Geometry: see drawing. Coordinates: mm, zero at the bounding-box minimum. A direction names the side the tool comes from. Give positions to 0.01 mm unless a question says otherwise; leave off trailing zeros. Order: outer loops, then holes, each group sorted by start corner. A loop starts at its lowest first (then second) coordinate and runs counter-clockwise, first axis right, second up. Notation, with made-up numbers: (-15.5, 67.25) - (15.5, 67.25) arc R19 ccw to (15.5, 87.25) - close; hole circle Ø3 at (22.5, 20). An arc over 180 degrees is marked (long way). One line per item, written item: value. Start each with the question number.
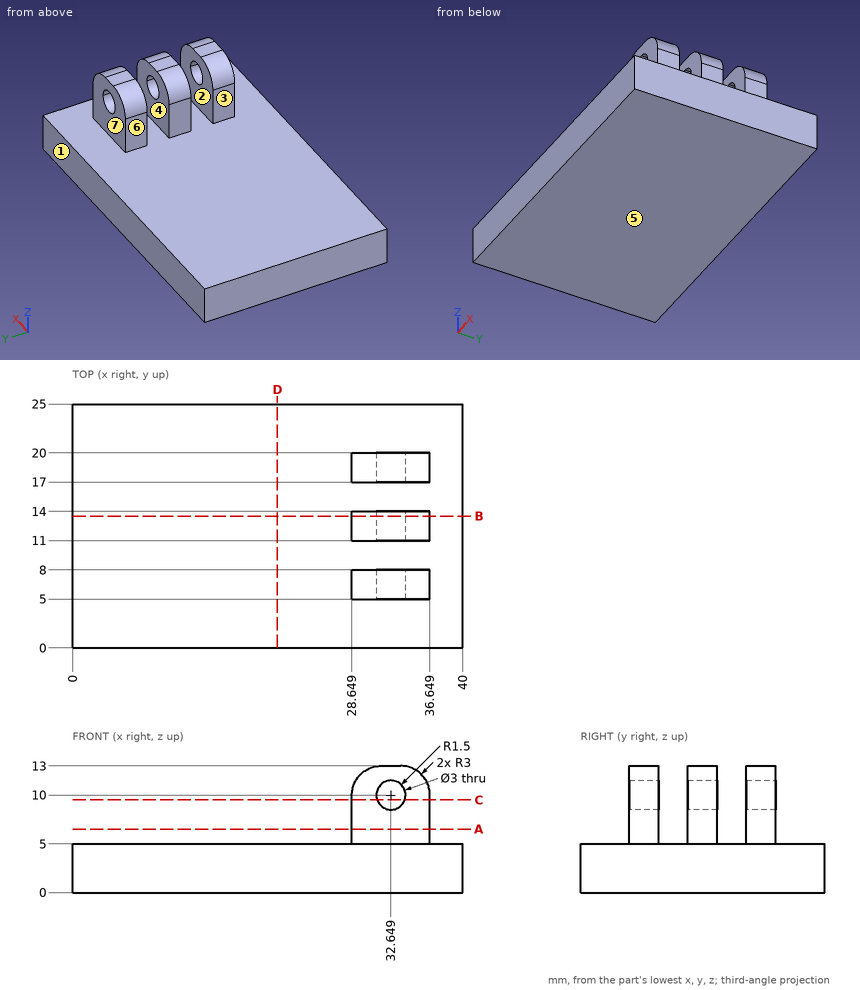
1. Draft query along Y for the marked faces 1, 2, 3 and 4. Return one class per face: pulls with the +Y half, pulls with the -Y half, needs draft (parallel to the pull), parting line crosses it, or undercut.
2. Section B-B on y = 13.5. Return the cut outline in (x, z), then the cut area to 3 significant figures.
3. Section D-D on x = 21. Return the cut outline in (y, z).
4. Contact query for flat-ended pins moving along their axis: pin 1 Ø0.9 at (y, z) = (13, 8.5) entering from +X; pin 2 Ø2.5 at (y, z) = (6.5, 7) entering from -X; pin 3 Ø8 at (x, y) = (14, 8) entering from +Z. Output: stop coordinate, or through.
5. Ray query, L1, parallel to Y at x = 36.5, z = 10.5; L2, parallel to X at y = 6.7, z = 10; L3, parallel to Z at x = 23, y = 23.25. Return the intervals inside material, ascending.
6. Section C-C on z = 9.5. Return the cut outline in (x, y) (1 decimal).
7. Section A-A on z = 6.5. Return the cut outline in (x, y), then the cut area to 3 significant figures.
8. Set-up query: the marked faces 5, 6 and 7. Return all of +Z, -Z, +X, -X, +Y, -Y with unobstructed straight access to the full face (end or side cutting, diameter ignored); none if empty.
Data:
1. face 1: pulls with the +Y half
1. face 2: undercut
1. face 3: needs draft
1. face 4: undercut
2. outline: (0, 0) - (40, 0) - (40, 5) - (36.65, 5) - (36.65, 10) arc R3 ccw to (33.65, 13) - (31.65, 13) arc R3 ccw to (28.65, 10) - (28.65, 5) - (0, 5) - close; hole circle Ø3 at (32.65, 10)
2. area: 253 mm2
3. outline: (0, 0) - (25, 0) - (25, 5) - (0, 5) - close
4. pin 1: stops at x = 36.65
4. pin 2: stops at x = 28.65
4. pin 3: stops at z = 5
5. L1: y = 5 to 8, 11 to 14, 17 to 20
5. L2: x = 28.65 to 31.15, 34.15 to 36.65
5. L3: z = 0 to 5
6. outline: (28.6, 5) - (31.2, 5) - (31.2, 8) - (28.6, 8) - close; (28.6, 11) - (31.2, 11) - (31.2, 14) - (28.6, 14) - close; (28.6, 17) - (31.2, 17) - (31.2, 20) - (28.6, 20) - close; (34.1, 5) - (36.6, 5) - (36.6, 8) - (34.1, 8) - close; (34.1, 11) - (36.6, 11) - (36.6, 14) - (34.1, 14) - close; (34.1, 17) - (36.6, 17) - (36.6, 20) - (34.1, 20) - close
7. outline: (28.65, 5) - (36.65, 5) - (36.65, 8) - (28.65, 8) - close; (28.65, 11) - (36.65, 11) - (36.65, 14) - (28.65, 14) - close; (28.65, 17) - (36.65, 17) - (36.65, 20) - (28.65, 20) - close
7. area: 72.0 mm2
8. face 5: -Z, +X, -X, +Y, -Y
8. face 6: +Z, -X, +Y, -Y
8. face 7: +Z, +X, -X, +Y
